from build123d import *

# Parameters (mm, degrees)
F0_R     = 21.85
F0_R_2   = 20.6
F0_R_3   = 15
F0_R_4   = 13.5
F1_DEPTH = 2
F2_DEPTH = 58
F3_SIZE  = 1


with BuildPart() as f1:
    # F0 (on Top) → F1 (new body)
    with BuildSketch(Plane.XY):
        Circle(F0_R)
        Circle(F0_R_2, mode=Mode.SUBTRACT)
        Circle(F0_R_2)
        Circle(F0_R_3, mode=Mode.SUBTRACT)
        Circle(F0_R_3)
        Circle(F0_R_4, mode=Mode.SUBTRACT)
    extrude(amount=F1_DEPTH)

    # F0 (on Top) → F2 (join)
    with BuildSketch(Plane.XY):
        Circle(F0_R_2)
        Circle(F0_R_3, mode=Mode.SUBTRACT)
        Circle(F0_R_3)
        Circle(F0_R_4, mode=Mode.SUBTRACT)
    extrude(amount=-F2_DEPTH)

    # F3
    f3_edges = [f1.edges().sort_by_distance(p)[0] for p in [
        (-20.6, 0, -58),
        (-13.5, 0, -58),
        (-13.5, 0, 2),
    ]]
    chamfer(f3_edges, length=F3_SIZE)


solid = f1.part
The listing builds one solid part. Answer for the finished solid, in the listing's coordinates (mm). A direction names the side the tool comes from. Give positions to 0.01 mm unless a question says otherwise; leave off trailing zeros. Order: outer loops, then holes, each group sorted by start corner. A loop starts at its lowest first (then second) coordinate and runs counter-clockwise, first axis right, second up. Notation, with made-up numbers: (66.5, 66.25) -> (102.5, 66.25) arc R17 ccw to (102.5, 90.25) -> close; hole circle Ø5 at (-21, 67). An arc over 180 degrees is marked (long way). Put each result on its own line as item: value.
Item 1: For faces 1 (the face through (19.65, 6.19, -28.1)), 2 (the face through (-4.74, -21.33, 0.99)), determine the directions among +Z, -Z, +X, -X, +Y, -Y from which every point of the face is accessible in a straight line to the end or side of a thin tool.
Established:
face 1: -Z
face 2: +Z, -Z
Item 2: Straight lines are drawn through the part: line 1 (Y direction, x = 0, z = 0.85); line 2 (Y direction, x = -2, z = -25); line 3 (X direction, y = -3, z = -38). For each, find the intervals that lie inside material, in ascending order.
Established:
line 1: y = -21.85 to -13.5, 13.5 to 21.85
line 2: y = -20.5 to -13.35, 13.35 to 20.5
line 3: x = -20.38 to -13.16, 13.16 to 20.38
Item 3: A cutting plane is placed at A-A on y = 0. Give the vertices of the cut face in (x, z), plus the area to 3 significant figures.
Established:
outline: (-21.85, 0) -> (-20.6, 0) -> (-20.6, -57) -> (-19.6, -58) -> (-14.5, -58) -> (-13.5, -57) -> (-13.5, 1) -> (-14.5, 2) -> (-21.85, 2) -> close; (13.5, -57) -> (14.5, -58) -> (19.6, -58) -> (20.6, -57) -> (20.6, 0) -> (21.85, 0) -> (21.85, 2) -> (14.5, 2) -> (13.5, 1) -> close
area: 854 mm^2
Item 4: Given P1, Ø5, axis at y = -12, z = -48, coming from the -X side; P2, Ø6, axis at x = -12, z = -17.5, coming from the -Y side; P3, Ø5, axis at x = 5, z = -28, coming from the -Y side; P4, Ø24.5, axis at x = 0, y = 0, coming from the +Z side, each flat-ended and moving along its own axis, determine where each tip first touches the part or whether it passes through.
Established:
P1: stops at x = -18.28
P2: stops at y = -18.53
P3: stops at y = -20.45
P4: passes through
Item 5: A cutting plane is placed at C-C on z = -17. Give the vertices of the cut face in (x, y).
Established:
outline: circle Ø41.2 at (0, 0); hole circle Ø27 at (0, 0)
